CAD build for the part. Positions are in the model's coordinates, mm. A direction names the side the tool comes from. Coordinates: 2 decimals unless noted, no trailing zeros. Loops run counter-clockwise (first coordinate to the right, second up) from the corner with the lowest first, then second, coordinate; pieces in that order, holes last. Notation, with made-up numbers: M 35.5,6.25 L 63.5,6.25 A15 cw 63.5,30.25 Z; hole C 32.5,70.5 d10. An arc over 180 degrees is marked long. Answer as a JSON object with one key per item and string values. Group by question number.
```python
from build123d import *

# Parameters (mm, degrees)
SKETCH_1_W      = 129
SKETCH_1_H      = 34
SKETCH_1_R      = 1.475
SKETCH_1_W_2    = 99
SKETCH_1_H_2    = 20
EXTRUDE_1_DEPTH = 3
FILLET_1_R      = 4


with BuildPart() as part:
    # 草图1 → 凸台-拉伸1 (new body)
    with BuildSketch(Plane.XY):
        Rectangle(SKETCH_1_W, SKETCH_1_H)
        with Locations((-57.5, 10)):
            Circle(SKETCH_1_R, mode=Mode.SUBTRACT)
        with Locations((-57.5, -10)):
            Circle(SKETCH_1_R, mode=Mode.SUBTRACT)
        with Locations(Location((57.5, -10, 0), (0, 0, 180))):
            Circle(SKETCH_1_R, mode=Mode.SUBTRACT)
        with Locations(Location((57.5, 10, 0), (0, 0, 180))):
            Circle(SKETCH_1_R, mode=Mode.SUBTRACT)
        Rectangle(SKETCH_1_W_2, SKETCH_1_H_2, mode=Mode.SUBTRACT)
    extrude(amount=EXTRUDE_1_DEPTH)

    # 圆角1
    fillet_1_edges = [part.edges().sort_by_distance(p)[0] for p in [
        (49.5, -10, 1.5),
        (49.5, 10, 1.5),
        (-49.5, 10, 1.5),
        (-49.5, -10, 1.5),
        (64.5, -17, 1.5),
        (-64.5, -17, 1.5),
        (-64.5, 17, 1.5),
        (64.5, 17, 1.5),
    ]]
    fillet(fillet_1_edges, radius=FILLET_1_R)


solid = part.part
```
Item 1: Slice it at B-B, the plane y = 1.5. Write the cut outline in (x, z).
Item 2: Slice it at A-A, the plane x = -57.5. Write the cut outline in (y, z) (3 decimals), then the cut area to 3 significant figures.
Item 3: Pull direction X, two halves, no side cores. Call faces 1 (the flat face through (-1, 12, 0)), 2 (the flat face through (-64.5, 0, 1)), 3 (the cylindrical face through (58.974, -10.065, 1.479)): released by +X, released by -X, zero draft, split by the parting line, or undercut.
Item 4: Slice it at C-C, the plane x = -21. Write the cut outline in (y, z), then the cut area to 3 significant figures.
Item 5: Pin check, flat tips, straight feed: pin 1 (12 mm diameter, centred on x = -41.5, y = 4.5, fed in from +Z); pin 2 (2.5 mm diameter, centred on x = -57.5, y = 10, fed in from +Z). Stop position of each tip, or through.
Item 6: Drill centre lines: L1, parallel to Y at x = 57.5, z = 2.05 (3 decimals); L2, parallel to Y at x = -15, z = 0.45; L3, parallel to X at y = -3, z = 2.2. Where is each one in solid material? Low to high. Write a range as from..to.
Item 7: Slice it at D-D, the plane z = 1.7. Write the cut outline in (x, y) (3 decimals), then the cut area to 3 significant figures.
Item 8: Tool access for faces 4 (the flat face through (-1, 17, 1)), 5 (the flat face through (49.5, 0, 1)): list every direction of +Z, -Z, +X, -X, +Y, -Y with a clear straight run to the whole face (end or side of a thin tool).
Computed:
{
 "1": {"outline": "M -64.5,0 L -49.5,0 L -49.5,3 L -64.5,3 Z; M 49.5,0 L 64.5,0 L 64.5,3 L 49.5,3 Z"},
 "2": {"outline": "M -17,0 L -11.475,0 L -11.475,3 L -17,3 Z; M -8.525,0 L 8.525,0 L 8.525,3 L -8.525,3 Z; M 11.475,0 L 17,0 L 17,3 L 11.475,3 Z", "area": "84.3 mm2"},
 "3": {"face 1": "zero draft", "face 2": "released by -X", "face 3": "undercut"},
 "4": {"outline": "M -17,0 L -10,0 L -10,3 L -17,3 Z; M 10,0 L 17,0 L 17,3 L 10,3 Z", "area": "42.0 mm2"},
 "5": {"pin 1": "z = 3", "pin 2": "through"},
 "6": {"L1": "-17..-11.475, -8.525..8.525, 11.475..17", "L2": "-17..-10, 10..17", "L3": "-64.5..-49.5, 49.5..64.5"},
 "7": {"outline": "M -64.5,-13 A4 ccw -60.5,-17 L 60.5,-17 A4 ccw 64.5,-13 L 64.5,13 A4 ccw 60.5,17 L -60.5,17 A4 ccw -64.5,13 Z; hole C -57.5,-10 d2.95; hole C -57.5,10 d2.95; hole M -49.5,-6 A4 ccw -45.5,-10 L 45.5,-10 A4 ccw 49.5,-6 L 49.5,6 A4 ccw 45.5,10 L -45.5,10 A4 ccw -49.5,6 Z; hole C 57.5,-10 d2.95; hole C 57.5,10 d2.95", "area": "2,380 mm2"},
 "8": {"face 4": "+Z, -Z, +X, -X, +Y", "face 5": "+Z, -Z"}
}
